```python
from build123d import *

# Parameters (mm, degrees)
SM_BASE_FLANGE_1_DEPTH             = 1.2
SKETCH_6_R                         = 2.5
CUT_EXTRUDE_1_DEPTH                = 10
SKETCH_7_R                         = 2
CUT_EXTRUDE_2_DEPTH                = 10
SKETCH_8_W                         = 3
SKETCH_8_H                         = 3
CUT_EXTRUDE_3_DEPTH                = 10
SM_EDGE_FLANGE_1_STRIP_W           = 6.2732
SM_EDGE_FLANGE_1_STRIP_H           = 1.2
SM_EDGE_FLANGE_1_STRIP_CUT_DEPTH   = 177
SM_EDGE_FLANGE_1_STRIP_2_W         = 6.2732
SM_EDGE_FLANGE_1_STRIP_2_H         = 1.2
SM_EDGE_FLANGE_1_STRIP_CUT_2_DEPTH = 180
SM_EDGE_FLANGE_1_DEPTH             = 177
SM_EDGE_FLANGE_1_BEND_DEPTH        = 180
CHAMFER_1_SIZE                     = 8


# Sheet-metal steps are written as plain solids
with BuildPart() as part:
    # Sketch 1 → Базовая кромка1 (new body)
    with BuildSketch(Plane.XY):
        Polygon((0, 270), (-21, 270), (-21, 348), (180, 348), (180, 0), (0, 0), align=None)
    extrude(amount=-SM_BASE_FLANGE_1_DEPTH)

    # Эскиз6 → Вырез-Вытянуть1 (cut)
    with BuildSketch(Plane.XY):
        with Locations((1, 309)):
            Circle(SKETCH_6_R)
    extrude(amount=-CUT_EXTRUDE_1_DEPTH, mode=Mode.SUBTRACT)

    # Эскиз7 → Вырез-Вытянуть2 (cut)
    with BuildSketch(Plane.XY):
        with Locations((171.5, 318)):
            Circle(SKETCH_7_R)
        with Locations((171.5, 303)):
            Circle(SKETCH_7_R)
        with Locations((171.5, 45)):
            Circle(SKETCH_7_R)
        with Locations((171.5, 30)):
            Circle(SKETCH_7_R)
    extrude(amount=-CUT_EXTRUDE_2_DEPTH, mode=Mode.SUBTRACT)

    # Эскиз8 → Вырез-Вытянуть3 (cut)
    with BuildSketch(Plane.XY):
        with Locations((1.5, 346.5)):
            Rectangle(SKETCH_8_W, SKETCH_8_H)
    extrude(amount=-CUT_EXTRUDE_3_DEPTH, mode=Mode.SUBTRACT)

    # Ребро-кромка1 strip (across the edge) → Ребро-кромка1 strip cut (cut)
    with BuildSketch(Plane(origin=(3, 348, -1.2), x_dir=(0, -1, 0), z_dir=(1, 0, 0))):
        with Locations((-1.2, -0.6)):
            Rectangle(SM_EDGE_FLANGE_1_STRIP_W, SM_EDGE_FLANGE_1_STRIP_H)
    extrude(amount=SM_EDGE_FLANGE_1_STRIP_CUT_DEPTH, mode=Mode.SUBTRACT)

    # Ребро-кромка1 strip 2 (across the edge) → Ребро-кромка1 strip cut 2 (cut)
    with BuildSketch(Plane(origin=(180, 0, -1.2), x_dir=(0, 1, 0), z_dir=(-1, 0, 0))):
        with Locations((-1.2, -0.6)):
            Rectangle(SM_EDGE_FLANGE_1_STRIP_2_W, SM_EDGE_FLANGE_1_STRIP_2_H)
    extrude(amount=SM_EDGE_FLANGE_1_STRIP_CUT_2_DEPTH, mode=Mode.SUBTRACT)

    # Ребро-кромка1 section (across the edge) → Ребро-кромка1 (add)
    with BuildSketch(Plane(origin=(3, 348, -1.2), x_dir=(0, -1, 0), z_dir=(1, 0, 0))):
        with BuildLine():
            Line((0, 0.7366), (0, 10.8))
            Line((0, 10.8), (1.2, 10.8))
            Line((1.2, 10.8), (1.2, 0.7366))
            ThreePointArc((1.2, 0.7366), (1.415745145, 0.215745145), (1.9366, 0))
            Line((1.9366, 0), (1.9366, -1.2))
            ThreePointArc((1.9366, -1.2), (0.567217008, -0.632782992), (0, 0.7366))
        make_face()
    extrude(amount=SM_EDGE_FLANGE_1_DEPTH)

    # Ребро-кромка1 section 2 (across the edge) → Ребро-кромка1 bend (add)
    with BuildSketch(Plane(origin=(180, 0, -1.2), x_dir=(0, 1, 0), z_dir=(-1, 0, 0))):
        with BuildLine():
            Line((0, 0.7366), (0, 10.8))
            Line((0, 10.8), (1.2, 10.8))
            Line((1.2, 10.8), (1.2, 0.7366))
            ThreePointArc((1.2, 0.7366), (1.415745145, 0.215745145), (1.9366, 0))
            Line((1.9366, 0), (1.9366, -1.2))
            ThreePointArc((1.9366, -1.2), (0.567217008, -0.632782992), (0, 0.7366))
        make_face()
    extrude(amount=SM_EDGE_FLANGE_1_BEND_DEPTH)

    # Фаска1
    chamfer_1_edges = [part.edges().sort_by_distance(p)[0] for p in [
        (3, 347.4, -12),
        (180, 347.4, -12),
        (180, 0.6, -12),
        (0, 0.6, -12),
    ]]
    chamfer(chamfer_1_edges, length=CHAMFER_1_SIZE)


solid = part.part
```
Input: part model. Units: mm. Frame: model coordinates. A direction names the side the tool comes from. Round coordinates to 2 decimals unless told otherwise and drop trailing zeros. Loops run counter-clockwise (first coordinate to the right, second up) from the corner with the lowest first, then second, coordinate; pieces in that order, holes last. Notation, with made-up numbers: (31.25, 57.5) - (63.25, 57.5) arc R17 ccw to (63.25, 85.5) - close; hole circle Ø5 at (13, -29). An arc over 180 degrees is marked (long way). One line per item, written item: value. Start each with the question number.
(1) Section A-A, the plane z = -6. Return loops of the section in (x, y), plus the area to 3 significant figures.
(2) Section C-C, the plane y = 156.5. Return loops of the section in (x, z).
(3) Access query for faces 1 (the flat face through (90, 346.8, -7)), 2 (the flat face through (7, 347, -8)), 3 (the flat face through (90, 348, -7)). Directions: +Z, -Z, +X, -X, +Y, -Y. A direction counts if a zero-diameter tool reaches every point of the face in a straight line with its end or side. Return the directions, or none.
(4) Draft query along Y for faces 4 (the flat face through (81, 177, -1.2)), 5 (the flat face through (91, 0, -7)), 6 (the flat face through (81, 177, 0)). Return one class per face: +Y half, -Y half, draft (parallel to the pull), parting line (faces both ways), or undercut.
(5) Section B-B, the plane x = 159. Return loops of the section in (y, z), plus the area to 3 significant figures.
(6) Contact query for flat-ended pins moving along their axis: P1, Ø3, axis at y = 171.5, z = -2, coming from the -X side; P2, Ø3, axis at x = 171.5, y = 303, coming from the +Z side; P3, Ø12, axis at x = 69, y = 175.5, coming from the -Z side; P4, Ø1, axis at x = 2, z = -1, coming from the +Y side. Output: stop coordinate, or through.
(7) Ray query, line 1 (Y direction, x = 65.5, z = -4.25); line 2 (Y direction, x = 171.5, z = -0.75); line 3 (X direction, y = 303, z = -0.4). Return the intervals inside material, ascending. Write a range as [from, to].
Results below:
1. outline: (2, 0) - (178, 0) - (178, 1.2) - (2, 1.2) - close; (5, 346.8) - (178, 346.8) - (178, 348) - (5, 348) - close
1. area: 419 mm^2
2. outline: (0, -1.2) - (180, -1.2) - (180, 0) - (0, 0) - close
3. face 1: -Z, +X, -X
3. face 2: -Z, -X, +Y
3. face 3: +Z, -Z, +X, -X, +Y
4. face 4: undercut
4. face 5: -Y half
4. face 6: draft
5. outline: (0, -12) - (1.2, -12) - (1.2, -1.94) arc R0.74 cw to (1.94, -1.2) - (346.06, -1.2) arc R0.74 cw to (346.8, -1.94) - (346.8, -12) - (348, -12) - (348, -1.94) arc R1.94 ccw to (346.06, 0) - (1.94, 0) arc R1.94 ccw to (0, -1.94) - close
5. area: 442 mm^2
6. P1: x = 0
6. P2: through
6. P3: z = -1.2
6. P4: y = 345
7. line 1: [0, 1.2], [346.8, 348]
7. line 2: [0.41, 28], [32, 43], [47, 301], [305, 316], [320, 347.59]
7. line 3: [-21, 169.5], [173.5, 180]
